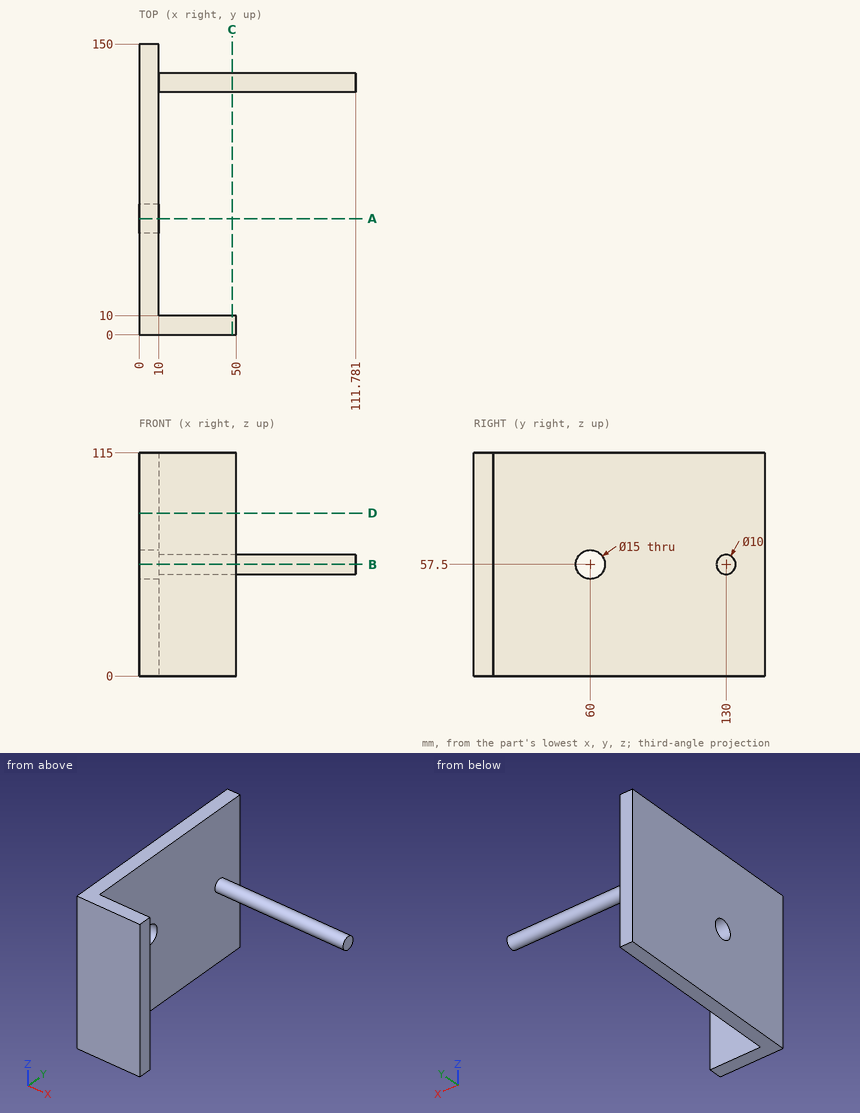
Design review of the part shown in the three views and the two pictorial views. Dimensions are in mm from the part's minimum x, y and z. Coordinates: 2 decimals unless noted, no trailing zeros. Loops run counter-clockwise (first coordinate to the right, second up) from the corner with the lowest first, then second, coordinate; pieces in that order, holes last. Notation, with made-up numbers: M 72.25,-15 L 87.25,-15 A29 ccw 87.25,20 Z; hole C 67,-38.5 d8. An arc over 180 degrees is marked long. Put each result on its own line as item: value. Start each with the question number.
Q1. Add section C-C (x = 48). Write out the cut boundary in (y, z).
Q2. Add section B-B (z = 57.5). Write out the cut boundary in (x, y), and give its area (3 significant figures).
Q3. Wall thickness on line 1 (Y direction, x = 3.5, z = 57.5); line 2 (X direction, y = 97, z = 84); line 3 (Y direction, x = 60.5, z = 62): over which ranges is each line inside the solid? List them lowest first.
Q4. Add section D-D (z = 84). Write out the cut boundary in (x, y).
Q5. Clearance check with flat-ended pins moving along their axes: pin 1 (1 mm diameter, centred on y = 37, z = 72.5, fed in from +X); pin 2 (5 mm diameter, centred on y = 6, z = 82.5, fed in from +X). State where each tip first meets the part, or that it passes through.
Q6. Add section A-A (y = 60). Write out the cut boundary in (x, z).
Answers:
1. outline: M 0,0 L 10,0 L 10,115 L 0,115 Z; C 130,57.5 d10
2. outline: M 0,0 L 50,0 L 50,10 L 10,10 L 10,52.5 L 0,52.5 Z; M 0,67.5 L 10,67.5 L 10,125 L 111.78,125 L 111.78,135 L 10,135 L 10,150 L 0,150 Z
2. area: 2,770 mm^2
3. line 1: y = 0 to 52.5, 67.5 to 150
3. line 2: x = 0 to 10
3. line 3: y = 127.82 to 132.18
4. outline: M 0,0 L 50,0 L 50,10 L 10,10 L 10,150 L 0,150 Z
5. pin 1: stops at x = 10
5. pin 2: stops at x = 50
6. outline: M 0,0 L 10,0 L 10,50 L 0,50 Z; M 0,65 L 10,65 L 10,115 L 0,115 Z
